Source: CAD feature listing. Evaluate the final solid. Frame: model axes, mm. A direction names the side the tool comes from. Give positions to 0.01 mm unless a question says otherwise; leave off trailing zeros. Loops run counter-clockwise (first coordinate to the right, second up) from the corner with the lowest first, then second, coordinate; pieces in that order, holes last. Notation, with made-up numbers: M 83,34.25 L 109,34.25 A33 ccw 109,65.25 Z; hole C 63,31.5 d11. An arc over 180 degrees is marked long. Write item = value, one per line.
from build123d import *

# Parameters (mm, degrees)
F0_R     = 9.5
F1_DEPTH = 6.8
F2_R     = 7
F3_DEPTH = 9
F5_DEPTH = 4.8
F6_R     = 3.35
F7_DEPTH = 15.801
F8_SIZE  = 0.5


with BuildPart() as f1:
    # F0 (on Top) → F1 (new body)
    with BuildSketch(Plane.XY):
        Circle(F0_R)
    extrude(amount=F1_DEPTH)

    # F2 (on face) → F3 (join)
    with BuildSketch(Plane.XY.offset(6.8)):
        Circle(F2_R)
    extrude(amount=F3_DEPTH)

    # F4 (on face) → F5 (cut)
    with BuildSketch(Plane(origin=(0, 0, 0), x_dir=(1, 0, 0), z_dir=(0, 0, -1))):
        Polygon((-5.15, -2.973354), (0, -5.946708), (5.15, -2.973354), (5.15, 2.973354), (0, 5.946708), (-5.15, 2.973354), align=None)
    extrude(amount=-F5_DEPTH, mode=Mode.SUBTRACT)

    # F6 (on face) → F7 (cut, through all)
    with BuildSketch(Plane.XY.offset(15.8)):
        Circle(F6_R)
    extrude(amount=-F7_DEPTH, mode=Mode.SUBTRACT)

    # F8
    f8_edges = [f1.edges().sort_by_distance(p)[0] for p in [
        (-7, 0, 15.8),
        (-3.35, 0, 15.8),
        (-9.5, 0, 0),
    ]]
    chamfer(f8_edges, length=F8_SIZE)


solid = f1.part
1. Pull-direction query (X, two-part tool) for faces 1 (the flat face through (2.61, -4.44, 2.37)), 2 (the flat face through (-2.54, -4.48, 2.37)), 3 (the cylindrical face through (4.38, -8.43, 3.61)), 4 (the flat face through (-4, -6, 6.8)); classes: +X half, -X half, draft (parallel to the pull), parting line (faces both ways), or undercut.
Derived:
face_1 = undercut
face_2 = undercut
face_3 = parting line
face_4 = draft
2. Reachability of faces 5 (the cylindrical face through (6.466, -2.681, 10.99)), 6 (the flat face through (5.15, 0, 2)), 7 (the flat face through (4, -4, 0)) from +Z, -Z, +X, -X, +Y, -Y: full face, straight path, thin tool, end or side. Return the list, or none.
Derived:
face_5 = +Z
face_6 = -Z
face_7 = -Z, +X, -X, +Y, -Y
3. Cut plane A-A, the plane y = 0. Return the cut outline in (x, z).
Derived:
outline = M -9.5,0.5 L -9,0 L -5.15,0 L -5.15,4.8 L -3.35,4.8 L -3.35,15.3 L -3.85,15.8 L -6.5,15.8 L -7,15.3 L -7,6.8 L -9.5,6.8 Z; M 3.35,4.8 L 5.15,4.8 L 5.15,0 L 9,0 L 9.5,0.5 L 9.5,6.8 L 7,6.8 L 7,15.3 L 6.5,15.8 L 3.85,15.8 L 3.35,15.3 Z
4. Material intervals for probe 1 along Y at (x, z) = (0, 11.75); probe 2 along Z at (x, y) = (4.5, -0.75); probe 3 along Y at (x, z) = (-1, 13.75), sorted ascending. Write a range as from..to.
Derived:
probe_1 = -7..-3.35, 3.35..7
probe_2 = 4.8..15.8
probe_3 = -6.93..-3.2, 3.2..6.93
5. First-contact query: pin 1 Ø3 at (x, y) = (2, -1.5) entering from -Z; pin 2 Ø8 at (x, z) = (-5, 8) entering from +Y; pin 3 Ø8 at (x, z) = (-7, 12) entering from -Y; pin 4 Ø6 at (x, y) = (0, 0) entering from -Z. Flat tips, straight axial feed; report the tip coordinate or a pass-through.
Derived:
pin_1 = 4.8
pin_2 = 9.43
pin_3 = -6.32
pin_4 = through
6. Cut plane B-B, the plane z = 14.75. Return the cut outline in (x, y).
Derived:
outline = C 0,0 d14; hole C 0,0 d6.7
